from build123d import *

# Parameters (mm, degrees)
F3_R      = 15
F4_DEPTH  = 5
F5_R      = 20
F9_R      = 11
F10_DEPTH = 30


with BuildPart() as f2:
    # F1 (on Front) → F2 (revolve)
    with BuildSketch(Plane.XZ):
        Polygon((150, 100), (150, 0), (167.5, 0), (167.5, 80), (202.5, 80), (202.5, 100), align=None)
    revolve(axis=Axis((150, 0, 50), (0, 0, 1)))



with BuildPart() as f4:
    # F3 (on Right) → F4 (new body, symmetric)
    with BuildSketch(Plane.YZ):
        Polygon((115, 0), (205, 0), (160, 65), align=None)
        with Locations((160, 25)):
            Circle(F3_R, mode=Mode.SUBTRACT)
    extrude(amount=F4_DEPTH, both=True)

    # F5
    f5_edges = [f4.edges().sort_by_distance(p)[0] for p in [
        (0, 160, 65),
    ]]
    fillet(f5_edges, radius=F5_R)


with BuildPart() as f6_1:
    # F6: instance of F4
    add(f4.part.mirror(Plane.XZ))


with BuildPart() as f8:
    # F7 (on Front) → F8 (revolve)
    with BuildSketch(Plane.XZ):
        Polygon((0, -235), (350, -235), (350, -170), (320, -170), (320, -215), (0, -215), align=None)
    revolve(axis=Axis((246.6098368168, 0, -310), (1, 0, 0)))

    # F9 (on face) → F10 (cut, through all)
    with BuildSketch(Plane.YZ.offset(350)):
        with Locations((0, -190)):
            Circle(F9_R)
    extrude(amount=-F10_DEPTH, mode=Mode.SUBTRACT)

    # F11: F8 across plane


with BuildPart() as f8_1:
    add(f8.part)
    add(f8.part.mirror(Plane.YZ))


with BuildPart() as f2_1:
    add(f2.part)

    add(f4.part)  # F12 merges F4

    add(f6_1.part)  # F12 merges F6_1

    add(f8_1.part)  # F12 merges F8
    # F0 (on Front) → F12 (revolve)
    with BuildSketch(Plane.XZ):
        Polygon((255, 0), (0, 0), (0, -650), (155, -650), (155, -80), (255, -80), align=None)
    revolve(axis=Axis((0, 0, 290.8246964216), (0, 0, 1)))


solid = f2_1.part
Geometry: final body of the model. Coordinates: model frame, mm. A direction names the side the tool comes from. Round coordinates to 2 decimals unless told otherwise and drop trailing zeros. Order: outer loops, then holes, each group sorted by start corner. A loop starts at its lowest first (then second) coordinate and runs counter-clockwise, first axis right, second up. Notation, with made-up numbers: (42.5, 26.5) -> (96.5, 26.5) arc R24 ccw to (96.5, 52.5) -> close; hole circle Ø6 at (5.5, 19). An arc over 180 degrees is marked (long way). Put each result on its own line as item: value. Start each with the question number.
Q1. Reachability of faces 1 (the flat face through (320, 91, -281)), 2 (the cylindrical face through (335.21, -1.432, -179.094)), 3 (the flat face through (5, 159, 9)), 4 (the flat face through (0.07, -129.478, 20.913)), 5 (the cylindrical face through (-334.79, 53.621, -180.676)) from +Z, -Z, +X, -X, +Y, -Y: full face, straight path, thin tool, end or side. Return the list, or none.
Q2. Section B-B on y = -125.5. Return the cut outline in (x, z), and give its area (3 significant figures).
Q3. First-contact query: pin 1 (1 mm diameter, centred on y = 103.5, z = -158, fed in from -X); pin 2 (25 mm diameter, centred on y = 181, z = 20, fed in from -X); pin 3 (2 mm diameter, centred on y = 106.5, z = -522.5, fed in from +X). Flat tips, straight axial feed; report the tip coordinate or a pass-through.
Q4. Section D-D on z = -310. Return the cut outline in (x, y), and give its area (3 significant figures).
Q5. Pull-direction query (X, two-part tool) for faces 6 (the flat face through (0.07, -190.92, 20.34)), 7 (the cylindrical face through (-123, -94.32, -361.01)), 8 (the flat face through (5, -159, 9)); classes: +X half, -X half, draft (parallel to the pull), parting line (faces both ways), or undercut.
Q6. Line query: probe 1 along Z at (x, y) = (-334, 0); probe 2 along Z at (x, y) = (303, 0); probe 3 along Z at (x, y) = (-2.5, 160). Output: solid intervals per line, ascending.
Q7. Section C-C on x = -180.5. Return the cut outline in (y, z).
Q8. Section A-A on z = 25. Return the cut outline in (x, y), and give its area (3 significant figures).
Ans:
1. face 1: none
1. face 2: +X
1. face 3: +Z, +X, +Y, -Y
1. face 4: +Z, +X, -X
1. face 5: -X
2. outline: (-350, -372.05) -> (-320, -372.05) -> (-320, -247.95) -> (-350, -247.95) -> close; (-221.98, -80) -> (-90.97, -80) -> (-90.97, -650) -> (90.97, -650) -> (90.97, -80) -> (221.98, -80) -> (221.98, 0) -> (5, 0) -> (5, 15.17) -> (-5, 15.17) -> (-5, 0) -> (-221.98, 0) -> close; (320, -372.05) -> (350, -372.05) -> (350, -247.95) -> (320, -247.95) -> close
2. area: 147,000 mm2
3. pin 1: stops at x = -115.83
3. pin 2: stops at x = -5
3. pin 3: stops at x = 113.56
4. outline: (-350, -140) -> (-320, -140) -> (-320, -95) -> (-122.47, -95) arc R155 ccw to (122.47, -95) -> (320, -95) -> (320, -140) -> (350, -140) -> (350, -75) -> (135.65, -75) arc R155 ccw to (135.65, 75) -> (350, 75) -> (350, 140) -> (320, 140) -> (320, 95) -> (122.47, 95) arc R155 ccw to (-122.47, 95) -> (-320, 95) -> (-320, 140) -> (-350, 140) -> (-350, 75) -> (-135.65, 75) arc R155 ccw to (-135.65, -75) -> (-350, -75) -> close
4. area: 98,500 mm2
5. face 6: draft
5. face 7: undercut
5. face 8: +X half
6. probe 1: z = -450 to -385, -235 to -201, -179 to -170
6. probe 2: z = -405 to -385, -235 to -215
6. probe 3: z = -80 to 10, 40 to 49.86
7. outline: (-180.12, -80) -> (180.12, -80) -> (180.12, 0) -> (-180.12, 0) -> close; circle Ø190 at (0, -310); hole circle Ø150 at (0, -310)
8. outline: (-5, -187.69) -> (5, -187.69) -> (5, -175) -> (-5, -175) -> close; (-5, -145) -> (5, -145) -> (5, -132.31) -> (-5, -132.31) -> close; (-5, 132.31) -> (5, 132.31) -> (5, 145) -> (-5, 145) -> close; (-5, 175) -> (5, 175) -> (5, 187.69) -> (-5, 187.69) -> close; circle Ø35 at (150, 0)
8. area: 1,470 mm2
